from build123d import *

# Parameters (mm, degrees)
SKETCH1_W               = 120
SKETCH1_H               = 137
BOSS_EXTRUDE1_DEPTH     = 3
SKETCH2_W               = 120
SKETCH2_H               = 5
BOSS_EXTRUDE2_DEPTH     = 8
SKETCH3_W               = 38
SKETCH3_H               = 10
CUT_EXTRUDE1_DEPTH      = 25
SKETCH4_W               = 120
SKETCH4_H               = 124
CUT_EXTRUDE2_DEPTH      = 92.412526494
CUT_EXTRUDE2_DEPTH_BACK = 92.412526494
BOSS_EXTRUDE3_DEPTH     = 7
BOSS_EXTRUDE4_DEPTH     = 120
SKETCH9_W               = 5
SKETCH9_H               = 23
CUT_EXTRUDE3_DEPTH      = 250
MOVE_FACE1_BY           = 5


with BuildPart() as part:
    # Sketch1 → Boss-Extrude1 (new body)
    with BuildSketch(Plane(origin=(0, 0, 0), x_dir=(1, 0, 0), z_dir=(0, 1, 0))):
        Rectangle(SKETCH1_W, SKETCH1_H)
    extrude(amount=BOSS_EXTRUDE1_DEPTH)

    # Sketch2 → Boss-Extrude2 (add)
    with BuildSketch(Plane(origin=(0, 3, 0), x_dir=(1, 0, 0), z_dir=(0, 1, 0))):
        with Locations((0, -66)):
            Rectangle(SKETCH2_W, SKETCH2_H)
    extrude(amount=BOSS_EXTRUDE2_DEPTH)

    # Sketch3 → Cut-Extrude1 (cut)
    with BuildSketch(Plane(origin=(0, 11, 0), x_dir=(1, 0, 0), z_dir=(0, 1, 0))):
        with Locations((0, -63.5)):
            Rectangle(SKETCH3_W, SKETCH3_H)
    extrude(amount=-CUT_EXTRUDE1_DEPTH, mode=Mode.SUBTRACT)

    # Sketch4 → Cut-Extrude2 (cut, two sides)
    with BuildSketch(Plane(origin=(0, 3, 0), x_dir=(1, 0, 0), z_dir=(0, 1, 0))) as cut_extrude2_sk:
        with Locations((0, 6.5)):
            Rectangle(SKETCH4_W, SKETCH4_H)
    extrude(amount=CUT_EXTRUDE2_DEPTH, mode=Mode.SUBTRACT)
    extrude(cut_extrude2_sk.sketch, amount=-CUT_EXTRUDE2_DEPTH_BACK, mode=Mode.SUBTRACT)

    # Sketch7 → Boss-Extrude3 (add)
    with BuildSketch(Plane.ZY.offset(60)):
        Polygon((63.5, 11), (63.5, 3), (55.5, 3), (55.5, 0), (68.5, 0), (68.5, 11), align=None)
    extrude(amount=BOSS_EXTRUDE3_DEPTH)

    # Sketch8 → Boss-Extrude4 (add)
    with BuildSketch(Plane(origin=(60, 0, 0), x_dir=(0, 0, -1), z_dir=(1, 0, 0))):
        Polygon((-55.5, 0), (-55.5, 3), (-63.5, 3), (-63.5, 11), (-68.5, 11), (-68.5, 1.6), (-86.5, 1.6), (-86.5, 11), (-91.5, 11), (-91.5, 0), align=None)
    extrude(amount=BOSS_EXTRUDE4_DEPTH)

    # Sketch9 → Cut-Extrude3 (cut)
    with BuildSketch(Plane(origin=(0, 11, 0), x_dir=(1, 0, 0), z_dir=(0, 1, 0))):
        with Locations((62.5, -80)):
            Rectangle(SKETCH9_W, SKETCH9_H)
    extrude(amount=-CUT_EXTRUDE3_DEPTH, mode=Mode.SUBTRACT)

    # Move Face1: a face moved inward by 5.0
    extrude(part.faces().sort_by_distance((180, 1.1, 73.5))[0], amount=MOVE_FACE1_BY, dir=(-1, 0, 0), mode=Mode.SUBTRACT)


solid = part.part
CAD build for the part. Positions are in the model's coordinates, mm. A direction names the side the tool comes from. Give positions to 0.01 mm unless a question says otherwise; leave off trailing zeros. Write each loop counter-clockwise with the first axis right and the second up, starting at its lowest first coordinate (ties: lowest second). Pieces come first, ordered by that corner, then holes. Notation, with made-up numbers: M -18,44 L 20,44 A29 ccw 20,71 Z; hole C -31.5,1 d6. An arc over 180 degrees is marked long. Put each result on its own line as item: value. Start each with the question number.
(1) Band-saw the part on D-D, the plane z = 75. Write the cut outline in (x, y).
(2) Flat gauge pins, fed straight in: pin 1 Ø6.5 at (x, y) = (115.5, 8.5) entering from -Z; pin 2 Ø5.5 at (y, z) = (3, 77.5) entering from -X; pin 3 Ø0.9 at (x, y) = (0, 2) entering from +Z; pin 4 Ø2 at (y, z) = (4, 74) entering from +X. Where does each tip first touch, or does it go through?
(3) Band-saw the part on C-C, the plane x = 82. Write the cut outline in (y, z), and give its area (3 significant figures).
(4) Mould opens along Z. For faces 1 (the face through (119, 6, 86.5)), 2 (the face through (119, 6, 91.5)), 3 (the face through (-19, 4, 65)), 4 (the face through (-43, 7, 63.5)) say: +Z half, -Z half, draft (parallel to the pull), parting line (faces both ways), or undercut.
(5) Which spindle directions (+Z, -Z, +X, -X, +Y, -Y) get a long thin tool onto all of the face, cutting with end or side? Do faces 5 (the face through (65, 4, 87)), 6 (the face through (119, 1.6, 77)), 7 (the face through (52, 3, 59)), 8 (the face through (19, 4, 65)). Say none if no direction does.
(6) Probe L1, parallel to Z at x = 69.5, y = 7.75; L2, parallel to Z at x = 163, y = 1.75; L3, parallel to X at y = 6, z = 65.5. List the from-to ranges inside material, lowest first.
(7) Band-saw the part on B-B, the plane z = 61.5. Write the cut outline in (x, y).
(8) Band-saw the part on A-A, the plane y = 7.25. Write the cut outline in (x, z), and give its area (3 significant figures).
Response values:
1. outline: M 65,0 L 175,0 L 175,1.6 L 65,1.6 Z
2. pin 1: stops at z = 63.5
2. pin 2: stops at x = 65
2. pin 3: stops at z = 58.5
2. pin 4: passes through
3. outline: M 0,55.5 L 3,55.5 L 3,63.5 L 11,63.5 L 11,68.5 L 1.6,68.5 L 1.6,86.5 L 11,86.5 L 11,91.5 L 0,91.5 Z
3. area: 163 mm2
4. face 1: undercut
4. face 2: +Z half
4. face 3: draft
4. face 4: -Z half
5. face 5: +Z, -X, +Y, -Y
5. face 6: +X, -X, +Y
5. face 7: -Z, +X, -X, +Y
5. face 8: +Z, +Y, -Y
6. L1: z = 63.5 to 68.5, 86.5 to 91.5
6. L2: z = 55.5 to 68.5, 86.5 to 91.5
6. L3: x = -67 to -19, 19 to 175
7. outline: M -67,0 L -19,0 L -19,3 L -67,3 Z; M 19,0 L 175,0 L 175,3 L 19,3 Z
8. outline: M -67,63.5 L -19,63.5 L -19,68.5 L -67,68.5 Z; M 19,63.5 L 175,63.5 L 175,68.5 L 19,68.5 Z; M 65,86.5 L 175,86.5 L 175,91.5 L 65,91.5 Z
8. area: 1,570 mm2
